Verification items for the finished model (mm, model axes). Face numbers are marked on the shaded views. A direction names the side the tool comes from. Coordinates: 2 decimals unless noted, no trailing zeros. Write each loop counter-clockwise with the first axis right and the second up, starting at its lowest first coordinate (ties: lowest second). Pieces come first, ordered by that corner, then holes. Notation, with made-up numbers: (-31.75, -31) -> (13.25, -31) arc R33 ccw to (13.25, 4) -> close; hole circle Ø1 at (71, -25.5). An arc over 180 degrees is marked (long way). Write each question's results on one line, items separated by ' | '. Start each with the question number.
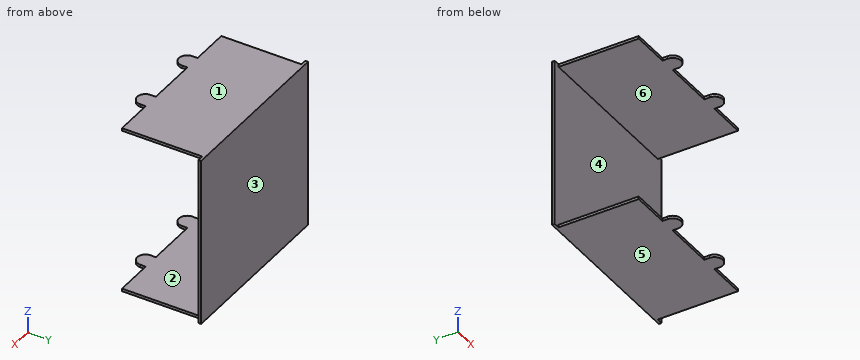
Autodesk Inventor part; units mm, degrees
ref_plane "shroud_to_body_XY" through (0, 0, 0) normal (0, 1, 0) x (1, 0, 0)
ref_plane "shroud_to_body_YZ" through (0, 0, 0) normal (1, 0, 0) x (0, 0, -1)
ref_plane "shroud_to_body_ZX" through (0, 0, 0) normal (0, 0, -1) x (0, 1, 0)
sketch "Sketch_1" plane through (0, 0, 0) normal (0, 1, 0) x (-1, 0, 0)
  line L0 (6.5024, 6.35) -> (-6.5024, 6.35)
  line L1 (-6.5024, 6.35) -> (-6.5024, -6.35)
  line L2 (-6.5024, -6.35) -> (6.5024, -6.35)
  line L3 (6.5024, -6.35) -> (6.5024, 6.35)
extrude "Extrusion1" add sketch "Sketch_1" along normal blind 0.2032
sketch "Sketch_2" plane through (0, 0, -6.35) normal (0, 0, 1) x (1, 0, 0)
  line L0 (-6.0389, -6.018) -> (-3.1581, -6.018)
  line L1 (-3.1581, -6.018) -> (-3.1581, -6.4159)
  arc A0 (-3.1581, -6.4159) -> (-1.9219, -6.4159) centre (-2.54, -6.4159) ccw
  line L2 (-1.9219, -6.4159) -> (-1.9219, -6.018)
  line L3 (-1.9219, -6.018) -> (1.9219, -6.018)
  line L4 (1.9219, -6.018) -> (1.9219, -6.4159)
  arc A1 (1.9219, -6.4159) -> (3.1581, -6.4159) centre (2.54, -6.4159) ccw
  line L5 (3.1581, -6.4159) -> (3.1581, -6.018)
  line L6 (3.1581, -6.018) -> (6.0389, -6.018)
  line L7 (6.0389, -6.018) -> (6.0389, 0)
  line L8 (6.0389, 0) -> (-6.0389, 0)
  line L9 (-6.0389, 0) -> (-6.0389, -6.018)
extrude "Extrusion2" add sketch "Sketch_2" along normal blind 0.2032
sketch "Sketch_3" plane through (0, 0, 6.35) normal (0, 0, 1) x (1, 0, 0)
  line L0 (-6.0389, -6.018) -> (-3.1581, -6.018)
  line L1 (-3.1581, -6.018) -> (-3.1581, -6.4159)
  arc A0 (-3.1581, -6.4159) -> (-1.9219, -6.4159) centre (-2.54, -6.4159) ccw
  line L2 (-1.9219, -6.4159) -> (-1.9219, -6.018)
  line L3 (-1.9219, -6.018) -> (1.9219, -6.018)
  line L4 (1.9219, -6.018) -> (1.9219, -6.4159)
  arc A1 (1.9219, -6.4159) -> (3.1581, -6.4159) centre (2.54, -6.4159) ccw
  line L5 (3.1581, -6.4159) -> (3.1581, -6.018)
  line L6 (3.1581, -6.018) -> (6.0389, -6.018)
  line L7 (6.0389, -6.018) -> (6.0389, 0)
  line L8 (6.0389, 0) -> (-6.0389, 0)
  line L9 (-6.0389, 0) -> (-6.0389, -6.018)
extrude "Extrusion3" add sketch "Sketch_3" against normal blind 0.2032
ref_plane "shroud_to_body_XY" through (0, 0, 0) normal (0, 1, 0) x (1, 0, 0)
ref_plane "shroud_to_body_YZ" through (0, 0, 0) normal (1, 0, 0) x (0, 0, -1)
ref_plane "shroud_to_body_ZX" through (0, 0, 0) normal (0, 0, -1) x (0, 1, 0)
properties part number "M20_ang_t_shorud2830TX-switch"
1. Tool access check on the marked faces 1 and 2. Record the directions out of +Z, -Z, +X, -X, +Y, -Y that give a thin tool (end or side, any length) a straight path to the whole face; none if there is none.
2. Sectioned sample at A-A on y = -5.5. Record the cut outline in (x, z), plus the area to 3 significant figures.
3. Material ranges on probe 1 along Z at (x, y) = (-1.75, -5); probe 2 along Y at (x, z) = (-1.5, -0.75), recorded low to high. Write a range as from..to.
4. Mould release check, pull along Z, two halves, no side actions. Record for the marked faces 3, 4, 5 and 6: +Z half, -Z half, draft (parallel to the pull), parting line (faces both ways), or undercut.
5. Sectioned sample at D-D on z = 2.5. Record the cut outline in (x, y), plus the area to 3 significant figures.
6. Depth check by flat-ended pin: pin 1 Ø5 at (x, z) = (1.5, -0.5) entering from -Y; pin 2 Ø2 at (y, z) = (-2.5, 2) entering from +X. Enter the tip coordinate at first touch or a pass-through.
7. Sectioned sample at B-B on y = -6.25. Record the cut outline in (x, z).
8. Sectioned sample at C-C on x = -5.25. Record the cut outline in (y, z), plus the area to 3 significant figures.
Computed values:
1) face 1: +Z, +X, -X, +Y, -Y | face 2: +X, -X, -Y
2) outline: (-6.04, -6.35) -> (6.04, -6.35) -> (6.04, -6.15) -> (-6.04, -6.15) -> close; (-6.04, 6.15) -> (6.04, 6.15) -> (6.04, 6.35) -> (-6.04, 6.35) -> close | area: 4.91 mm^2
3) probe 1: z = -6.35..-6.15, 6.15..6.35 | probe 2: y = 0..0.2
4) face 3: draft | face 4: undercut | face 5: -Z half | face 6: undercut
5) outline: (-6.5, 0) -> (6.5, 0) -> (6.5, 0.2) -> (-6.5, 0.2) -> close | area: 2.64 mm^2
6) pin 1: stops at y = 0 | pin 2: passes through
7) outline: (-3.16, -6.35) -> (-1.92, -6.35) -> (-1.92, -6.15) -> (-3.16, -6.15) -> close; (-3.16, 6.15) -> (-1.92, 6.15) -> (-1.92, 6.35) -> (-3.16, 6.35) -> close; (1.92, -6.35) -> (3.16, -6.35) -> (3.16, -6.15) -> (1.92, -6.15) -> close; (1.92, 6.15) -> (3.16, 6.15) -> (3.16, 6.35) -> (1.92, 6.35) -> close
8) outline: (-6.02, -6.35) -> (0.2, -6.35) -> (0.2, 6.35) -> (-6.02, 6.35) -> (-6.02, 6.15) -> (0, 6.15) -> (0, -6.15) -> (-6.02, -6.15) -> close | area: 5.03 mm^2
